Source: CAD feature listing. Evaluate the final solid. Frame: model axes, mm. Face numbers are marked on the shaded views. A direction names the side the tool comes from. Round coordinates to 2 decimals unless told otherwise and drop trailing zeros. Write each loop counter-clockwise with the first axis right and the second up, starting at its lowest first coordinate (ties: lowest second). Pieces come first, ordered by that corner, then holes.
```python
from build123d import *

# Parameters (mm, degrees)
SKETCH1_W           = 18.923
SKETCH1_H           = 22.606
BOSS_EXTRUDE1_DEPTH = 36.957
SKETCH2_R           = 10.9855
BOSS_EXTRUDE2_DEPTH = 28.0162
SKETCH3_W           = 2.794
SKETCH3_H           = 5.08
BOSS_EXTRUDE3_DEPTH = 5.08
SKETCH4_R           = 2.6924
BOSS_EXTRUDE4_DEPTH = 8.89


with BuildPart() as part:
    # Sketch1 → Boss-Extrude1 (new body)
    with BuildSketch(Plane.XY):
        with Locations((9.4615, 11.303)):
            Rectangle(SKETCH1_W, SKETCH1_H)
    extrude(amount=BOSS_EXTRUDE1_DEPTH)

    # Sketch2 → Boss-Extrude2 (add)
    with BuildSketch(Plane.XY.offset(36.957)):
        with Locations(Location((9.4615, 11.303, 0), (0, 0, 149.45966787))):
            Circle(SKETCH2_R)
    extrude(amount=BOSS_EXTRUDE2_DEPTH)

    # Sketch3 → Boss-Extrude3 (add)
    with BuildSketch(Plane(origin=(0, 0, 0), x_dir=(-1, 0, 0), z_dir=(0, 0, -1))):
        with Locations((-9.4615, 11.303)):
            Rectangle(SKETCH3_W, SKETCH3_H)
    extrude(amount=BOSS_EXTRUDE3_DEPTH)

    # Sketch4 → Boss-Extrude4 (add)
    with BuildSketch(Plane(origin=(18.923, 0, 0), x_dir=(0, 0, -1), z_dir=(1, 0, 0))):
        with Locations(Location((-10.8966, 10.8966, 0), (0, 0, 180))):
            Circle(SKETCH4_R)
    boss_extrude4 = extrude(amount=BOSS_EXTRUDE4_DEPTH)

    # Mirror1: Boss-Extrude4 across plane
    add(boss_extrude4.mirror(Plane(origin=(9.4615, 0, 0), x_dir=(0, 0, 1), z_dir=(1, 0, 0))))


solid = part.part
```
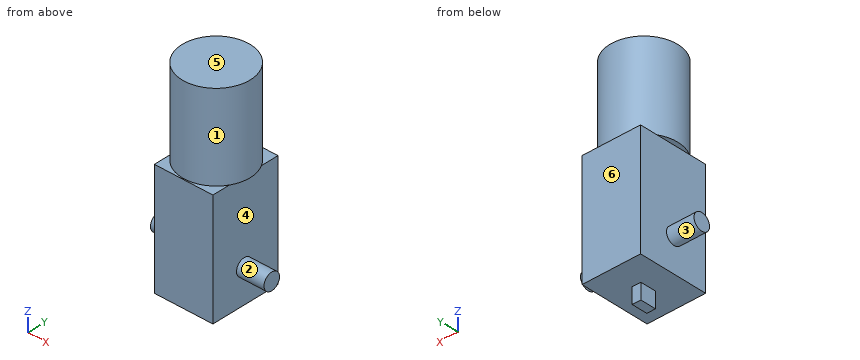
Q1. Section query D-D, the plane y = 3. Output: boundary loops of the cut face in (x, z).
Q2. Set-up query: the marked faces 1, 2 and 3. Return all of +Z, -Z, +X, -X, +Y, -Y with unobstructed straight access to the full face (end or side cutting, diameter ignored); none if empty.
Q3. Section query C-C, the plane x = 5. Output: boundary loops of the cut face in (y, z), and give its area (3 significant figures).
Q4. Section query A-A, the plane y = 12.5. Output: boundary loops of the cut face in (x, z).
Q5. Mould query, pull axis Z, two halves, no side actions, for the marked faces 4, 5 and 6. Classes: pulls with the +Z half, pulls with the -Z half, needs draft (parallel to the pull), parting line crosses it, or undercut.
Q6. Line query: line 1 (X direction, y = 11.5, z = 32.5); line 2 (Z direction, x = 18, y = 9.5); line 3 (Z direction, x = 0.5, y = 20). Output: solid intervals per line, ascending.
Q7. Pin query (flat end, axial travel): P1, Ø4, axis at y = 20, z = 50.5, coming from the -X side; P2, Ø11.5, axis at y = 13.5, z = 24.5, coming from the +X side; P3, Ø8, axis at x = 9.5, z = 58, coming from the -Y side; P4, Ø10, axis at x = 13, y = 8.5, coming from the -Z side. Return the tip coordinate at first contact, or that it passes through.
Q8. Section query B-B, the plane z = 23. Output: boundary loops of the cut face in (x, y).
Filled in:
1. outline: (0, 0) - (18.92, 0) - (18.92, 36.96) - (16.65, 36.96) - (16.65, 64.97) - (2.27, 64.97) - (2.27, 36.96) - (0, 36.96) - close
2. face 1: +Z
2. face 2: +X
2. face 3: -X
3. outline: (0, 0) - (22.61, 0) - (22.61, 36.96) - (21.34, 36.96) - (21.34, 64.97) - (1.26, 64.97) - (1.26, 36.96) - (0, 36.96) - close
3. area: 1,400 mm2
4. outline: (-8.89, 8.73) - (0, 8.73) - (0, 0) - (8.06, 0) - (8.06, -5.08) - (10.86, -5.08) - (10.86, 0) - (18.92, 0) - (18.92, 8.73) - (27.81, 8.73) - (27.81, 13.06) - (18.92, 13.06) - (18.92, 36.96) - (20.38, 36.96) - (20.38, 64.97) - (-1.46, 64.97) - (-1.46, 36.96) - (0, 36.96) - (0, 13.06) - (-8.89, 13.06) - close
5. face 4: undercut
5. face 5: pulls with the +Z half
5. face 6: needs draft
6. line 1: x = 0 to 18.92
6. line 2: z = 0 to 64.97
6. line 3: z = 0 to 36.96
7. P1: stops at x = 0.75
7. P2: stops at x = 18.92
7. P3: stops at y = 0.32
7. P4: stops at z = -5.08
8. outline: (0, 0) - (18.92, 0) - (18.92, 22.61) - (0, 22.61) - close
